Check sheet for the modelled part. Datum: model origin and axes. Units: mm. A direction names the side the tool comes from. Give positions to 0.01 mm unless a question says otherwise; leave off trailing zeros. Order: outer loops, then holes, each group sorted by start corner. A loop starts at its lowest first (then second) coordinate and runs counter-clockwise, first axis right, second up. Notation, with made-up numbers: (-13.5, -9.75) -> (32.5, -9.75) arc R31 cw to (32.5, 22.25) -> close; hole circle Ø8 at (-24.75, 60). An arc over 180 degrees is marked (long way). One line per question, with ' | ' between items.
```python
from build123d import *

# Parameters (mm, degrees)
SKETCH1_W                    = 100
SKETCH1_H                    = 60
BOSS_EXTRUDE1_DEPTH          = 1.6
SKETCH2_W                    = 28.451906957
SKETCH2_H                    = 12
BOSS_EXTRUDE2_DEPTH          = 4.5
SKETCH3_W                    = 21.668043294
SKETCH3_H                    = 24.059695689
BOSS_EXTRUDE3_DEPTH          = 1.27
F_3_0_3_DIAMETER_HOLE1_D     = 3
F_3_0_3_DIAMETER_HOLE1_DEPTH = 3.1496
F_3_0_3_DIAMETER_HOLE1_TIP   = 0.901290929


with BuildPart() as part:
    # Sketch1 → Boss-Extrude1 (new body)
    with BuildSketch(Plane.XY):
        Rectangle(SKETCH1_W, SKETCH1_H)
    extrude(amount=BOSS_EXTRUDE1_DEPTH)

    # Sketch2 → Boss-Extrude2 (add)
    with BuildSketch(Plane.XY.offset(1.6)):
        with Locations((-49.589851522, -1.044)):
            Rectangle(SKETCH2_W, SKETCH2_H)
    extrude(amount=BOSS_EXTRUDE2_DEPTH)

    # Sketch3 → Boss-Extrude3 (add)
    with BuildSketch(Plane.XY.offset(1.6)):
        with Locations((8.993071996, -8.71181328)):
            Rectangle(SKETCH3_W, SKETCH3_H)
    extrude(amount=BOSS_EXTRUDE3_DEPTH)

    # Ø3.0 (3) Diameter Hole1
    with Locations(Plane.XY.offset(1.6)):
        with Locations((-46.15, -26.15), (-46.15, 26.15), (46.15, -26.15), (46.15, 26.15)):
            Hole(F_3_0_3_DIAMETER_HOLE1_D / 2, depth=F_3_0_3_DIAMETER_HOLE1_DEPTH)
            with Locations((0, 0, -(F_3_0_3_DIAMETER_HOLE1_DEPTH + F_3_0_3_DIAMETER_HOLE1_TIP / 2))):  # 118° drill point
                Cone(0, F_3_0_3_DIAMETER_HOLE1_D / 2, F_3_0_3_DIAMETER_HOLE1_TIP, mode=Mode.SUBTRACT)


solid = part.part
```
Q1. Access from +Z, -Z, +X, -X, +Y, -Y to the whole of each face (thin tool, end or side, straight path). Record for faces 1 (the face through (-57, -1, 1.6)), 2 (the face through (-50, -7.044, 4)), 3 (the face through (9, -9, 2.87)), 4 (the face through (-50, -1, 6.1)).
Result sheet:
face 1: -Z, -X, +Y, -Y | face 2: +Z, -X, -Y | face 3: +Z, +X, +Y, -Y | face 4: +Z, +X, -X, +Y, -Y
Q2. Mould release check, pull along Y, two halves, no side actions. Record for faces 5 (the face through (-50, 4.956, 4)), 6 (the face through (-35.364, -1, 4)), 7 (the face through (-47.536, -26.725, 0.789)), 8 (the face through (47.34, -27.06, 0.79)): pulls with the +Y half, pulls with the -Y half, needs draft (parallel to the pull), parting line crosses it, or undercut.
Result sheet:
face 5: pulls with the +Y half | face 6: needs draft | face 7: undercut | face 8: undercut
Q3. Section check C-C (y = -9.5). Enter the section's corners in (x, z), and give its area (3 significant figures).
Result sheet:
outline: (-50, 0) -> (50, 0) -> (50, 1.6) -> (19.83, 1.6) -> (19.83, 2.87) -> (-1.84, 2.87) -> (-1.84, 1.6) -> (-50, 1.6) -> close | area: 188 mm2
Q4. Depth check by flat-ended pin: pin 1 Ø17.5 at (x, y) = (12.5, -7.5) entering from +Z; pin 2 Ø12 at (x, y) = (-24, -23) entering from +Z; pin 3 Ø1.3 at (x, z) = (-54.5, 4) entering from +Y; pin 4 Ø2.5 at (x, y) = (-46.15, -26.15) entering from +Z (3 decimals). Enter the tip coordinate at first touch or a pass-through.
Result sheet:
pin 1: stops at z = 2.87 | pin 2: stops at z = 1.6 | pin 3: stops at y = 4.96 | pin 4: passes through
Q5. Section check B-B (y = 26.15). Enter the section's corners in (x, z).
Result sheet:
outline: (-50, 0) -> (-47.65, 0) -> (-47.65, 1.6) -> (-50, 1.6) -> close; (-44.65, 0) -> (44.65, 0) -> (44.65, 1.6) -> (-44.65, 1.6) -> close; (47.65, 0) -> (50, 0) -> (50, 1.6) -> (47.65, 1.6) -> close
Q6. Section check A-A (x = 46.15). Enter the section's corners in (y, z).
Result sheet:
outline: (-30, 0) -> (-27.65, 0) -> (-27.65, 1.6) -> (-30, 1.6) -> close; (-24.65, 0) -> (24.65, 0) -> (24.65, 1.6) -> (-24.65, 1.6) -> close; (27.65, 0) -> (30, 0) -> (30, 1.6) -> (27.65, 1.6) -> close
Q7. Thickness scan on line 1 (Y direction, x = 46.15, z = 1.05); line 2 (Z direction, x = -32.5, y = 6); line 3 (Y direction, x = -37, z = 6). Record the ranges inside material, lowest first.
Result sheet:
line 1: y = -30 to -27.65, -24.65 to 24.65, 27.65 to 30 | line 2: z = 0 to 1.6 | line 3: y = -7.04 to 4.96
Q8. Section check D-D (x = 17.5). Enter the section's corners in (y, z).
Result sheet:
outline: (-30, 0) -> (30, 0) -> (30, 1.6) -> (3.32, 1.6) -> (3.32, 2.87) -> (-20.74, 2.87) -> (-20.74, 1.6) -> (-30, 1.6) -> close
